Here's how the part is built. I have some questions about the finished solid (model axes, mm). Round coordinates to 2 decimals unless told otherwise and drop trailing zeros. Loops run counter-clockwise (first coordinate to the right, second up) from the corner with the lowest first, then second, coordinate; pieces in that order, holes last. Notation, with made-up numbers: M -11.75,-24.75 L 40.25,-24.75 A14 ccw 40.25,-13.75 Z; hole C 0.25,-16.75 d10. An arc over 180 degrees is marked long. Answer as a JSON object with one key per item and string values.
from build123d import *

# Parameters (mm, degrees)
SKETCH1_R           = 25.5
SKETCH1_R_2         = 25
BOSS_EXTRUDE2_DEPTH = 10
BOSS_EXTRUDE3_START = -10
SKETCH1_4_R         = 28.5
SKETCH1_4_R_2       = 25.5
SKETCH1_4_R_3       = 25
BOSS_EXTRUDE3_DEPTH = 10
FILLET1_R           = 16


with BuildPart() as part:
    # Sketch1 → Boss-Extrude2 (new body)
    with BuildSketch(Plane(origin=(0, 0, 0), x_dir=(1, 0, 0), z_dir=(0, 1, 0))):
        with Locations(Location((0, 0, 0), (0, 0, 270))):
            Circle(SKETCH1_R)
        with Locations(Location((0, 0, 0), (0, 0, 270))):
            Circle(SKETCH1_R_2, mode=Mode.SUBTRACT)
    extrude(amount=BOSS_EXTRUDE2_DEPTH)

    # Sketch1<4> → Boss-Extrude3 (add)
    # profile 1 of 2: a face of its own
    with BuildSketch(Plane(origin=(0, 0, 0), x_dir=(1, 0, 0), z_dir=(0, 1, 0)).offset(BOSS_EXTRUDE3_START)):
        with Locations(Location((0, 0, 0), (0, 0, 270))):
            Circle(SKETCH1_4_R)
        with Locations(Location((0, 0, 0), (0, 0, 270))):
            Circle(SKETCH1_4_R_2, mode=Mode.SUBTRACT)
    # profile 2 of 2: a face of its own
    with BuildSketch(Plane(origin=(0, 0, 0), x_dir=(1, 0, 0), z_dir=(0, 1, 0)).offset(BOSS_EXTRUDE3_START)):
        with Locations(Location((0, 0, 0), (0, 0, 270))):
            Circle(SKETCH1_4_R_2)
        with Locations(Location((0, 0, 0), (0, 0, 270))):
            Circle(SKETCH1_4_R_3, mode=Mode.SUBTRACT)
    extrude(amount=BOSS_EXTRUDE3_DEPTH)

    # Chamfer1: read off the stored shape, not the designer's step
    # Chamfer1 outline → Chamfer1 (revolve, cut)
    with BuildSketch(Plane.XY):
        Polygon((28.5, -6.5), (25, -10), (28.5, -10), align=None)
    revolve(axis=Axis((0, 0, 0), (0, 1, 0)), mode=Mode.SUBTRACT)

    # Fillet1
    # the kernel refuses this fillet: 16 mm, written as the material it takes off along each edge
    with BuildSketch(Plane(origin=(0, -6.5, 0), x_dir=(0, 0, 1), z_dir=(-1, 0, 0))) as fillet1_piece_1:
        with BuildLine():
            CenterArc((12.5, 6.487492178), FILLET1_R, 321.375167127, 38.624832873)
            Line((25, -3.5), (28.5, 0))
            Line((28.5, 0), (28.5, 6.487492178))
        make_face()
    revolve(axis=Axis((0, -6.5, 0), (0, 1, 0)), revolution_arc=90, mode=Mode.SUBTRACT)
    with BuildSketch(Plane(origin=(0, -6.5, 0), x_dir=(1, 0, 0), z_dir=(0, 0, 1))) as fillet1_piece_2:
        with BuildLine():
            CenterArc((12.5, 6.487492178), FILLET1_R, 321.375167127, 38.624832873)
            Line((25, -3.5), (28.5, 0))
            Line((28.5, 0), (28.5, 6.487492178))
        make_face()
    revolve(axis=Axis((0, -6.5, 0), (0, 1, 0)), revolution_arc=270, mode=Mode.SUBTRACT)


solid = part.part
Item 1: Please list where these lines run through material, in increasing order: probe 1 along X at (y, z) = (1.5, 0); probe 2 along X at (y, z) = (-7, 2); probe 3 along Z at (x, y) = (9.5, -1). Write a range as from..to.
Resolved:
{"probe 1": "-25.5..-25, 25..25.5", "probe 2": "-26.82..-24.92, 24.92..26.82", "probe 3": "-26.84..-23.12, 23.12..26.84"}
Item 2: If we mould it in two halves opening along X, with no side actions, what happens to faces 1 (the face through (7.509, -0.14, 23.846)), 2 (the face through (-24.9, 4.9, -5.5)), 3 (the face through (-15, 0, -21))? For each: pulls with the +X half, pulls with the -X half, needs draft (parallel to the pull), parting line crosses it, or undercut.
Resolved:
{"face 1": "undercut", "face 2": "parting line crosses it", "face 3": "needs draft"}
Item 3: I want a section at A-A, the plane y = 1.25. Please give me the cut outline in (x, z), then the cut area to 3 significant figures.
Resolved:
{"outline": "C 0,0 d51; hole C 0,0 d50", "area": "79.3 mm²"}
Item 4: I'm going to push flat-ended pins straight in: pin 1 Ø4 at (x, y) = (-12.5, -2.5) entering from -Z; pin 2 Ø4 at (x, y) = (15.5, 6.5) entering from -Z; pin 3 Ø5 at (x, y) = (3, 6.5) entering from +Z. Where does each tip first touch, or does it pass through?
Resolved:
{"pin 1": "z = -26.34", "pin 2": "z = -21.63", "pin 3": "z = 25.5"}
